Check sheet for the modelled part. Datum: model origin and axes. Units: mm. Round coordinates to 2 decimals unless told otherwise and drop trailing zeros. Order: outer loops, then holes, each group sorted by start corner. A loop starts at its lowest first (then second) coordinate and runs counter-clockwise, first axis right, second up. Notation, with made-up numbers: (84, 85) -> (136, 85) arc R10 cw to (136, 99) -> close; hole circle Ø11 at (67, 28). An arc over 180 degrees is marked (long way). Answer in a Markdown table with one row per item. Add a question column.
1. Sectioned sample at A-A, the plane y = 3.5. Record the boundary of the cut face in (x, z).
2. Material ranges on L1, parallel to X at y = 11.25, z = 373.5; L2, parallel to Z at x = 161, y = 6.5; L3, parallel to Z at x = 152, y = 1.5, recorded low to high. Write a range as from..to.
3. Sectioned sample at B-B, the plane z = 244.5. Record the boundary of the cut face in (x, y), then the cut area to 3 significant figures.
4. Depth check by flat-ended pin: P1, Ø2, axis at x = 248.5, y = 6.5, coming from the +Z side; P2, Ø5, axis at x = 174, y = 8, coming from the +Z side. Enter the tip coordinate at first touch or a pass-through.
5. Sectioned sample at C-C, the plane x = 223.5. Record the boundary of the cut face in (y, z), then the cut area to 3 significant figures.
```python
from build123d import *

# Parameters (mm, degrees)
PAD_DEPTH = 13


with BuildPart() as part:
    # Sketch → Pad (new body)
    with BuildSketch(Plane.XZ):
        Polygon((0, 0), (280, 0), (280, 449.090952), (140.12854, 500), (0, 115), align=None)
    extrude(amount=-PAD_DEPTH)


solid = part.part
```
Answer key:
| question | item | result |
|---|---|---|
| 1 | outline | (0, 0) -> (280, 0) -> (280, 449.09) -> (140.13, 500) -> (0, 115) -> close |
| 2 | L1 | x = 94.09..280 |
| 2 | L2 | z = 0..492.4 |
| 2 | L3 | z = 0..495.68 |
| 3 | outline | (47.13, 0) -> (280, 0) -> (280, 13) -> (47.13, 13) -> close |
| 3 | area | 3,030 mm² |
| 4 | P1 | stops at z = 460.92 |
| 4 | P2 | stops at z = 488.58 |
| 5 | outline | (0, 0) -> (13, 0) -> (13, 469.66) -> (0, 469.66) -> close |
| 5 | area | 6,110 mm² |
